Verification items for the finished model (mm, model axes). A direction names the side the tool comes from. Coordinates: 2 decimals unless noted, no trailing zeros. Loops run counter-clockwise (first coordinate to the right, second up) from the corner with the lowest first, then second, coordinate; pieces in that order, holes last. Notation, with made-up numbers: (83, 36.25) -> (137, 36.25) arc R12 cw to (137, 49.25) -> close; hole circle Ø7 at (-3.5, -17.5). An arc over 180 degrees is marked (long way). Use CSV: the item, a comma, the result in double quotes. Start each with the question number.
```python
from build123d import *

# Parameters (mm, degrees)
SKETCH1_R                = 75
BOSS_EXTRUDE1_DEPTH      = 100
SKETCH5_R                = 29
CUT_EXTRUDE2_DEPTH       = 7
BOSS_EXTRUDE2_DEPTH      = 60
BOSS_EXTRUDE2_DEPTH_BACK = 60
SKETCH8_W                = 220
SKETCH8_H                = 180
BOSS_EXTRUDE3_DEPTH      = 10
SKETCH9_R                = 5
CUT_EXTRUDE4_DEPTH       = 10
FILLET1_R                = 10
SKETCH14_R               = 6
CUT_EXTRUDE6_DEPTH       = 110
SKETCH15_R               = 18.5
CUT_EXTRUDE7_DEPTH       = 97
SKETCH16_R               = 1.5
CUT_EXTRUDE8_DEPTH       = 7
SKETCH17_R               = 55
CUT_EXTRUDE9_DEPTH       = 73
SKETCH21_W               = 60
SKETCH21_H               = 80
CUT_EXTRUDE10_DEPTH      = 73
SKETCH23_R               = 2.75
CUT_EXTRUDE11_DEPTH      = 3
CUT_EXTRUDE15_DEPTH      = 40
CUT_EXTRUDE15_DEPTH_BACK = 40


with BuildPart() as part:
    # Sketch1 → Boss-Extrude1 (new body)
    with BuildSketch(Plane(origin=(0, 0, 0), x_dir=(1, 0, 0), z_dir=(0, 1, 0))):
        with Locations(Location((0, 0, 0), (0, 0, 270))):
            Circle(SKETCH1_R)
    extrude(amount=BOSS_EXTRUDE1_DEPTH)

    # Sketch5 → Cut-Extrude2 (cut)
    with BuildSketch(Plane(origin=(0, 100, 0), x_dir=(1, 0, 0), z_dir=(0, 1, 0))):
        with Locations(Location((0, 0, 0), (0, 0, 270))):
            Circle(SKETCH5_R)
    extrude(amount=-CUT_EXTRUDE2_DEPTH, mode=Mode.SUBTRACT)

    # Sketch2 → Boss-Extrude2 (add, two sides: drawn at the far end of the back side and taken through both)
    with BuildSketch(Plane.XY.offset(-BOSS_EXTRUDE2_DEPTH_BACK)):
        Polygon((0, 0), (-125, 0), (-90, 80), (0, 80), align=None)
    extrude(amount=BOSS_EXTRUDE2_DEPTH + BOSS_EXTRUDE2_DEPTH_BACK)

    # Sketch8 → Boss-Extrude3 (add)
    with BuildSketch(Plane.XZ):
        with Locations((-25, 0)):
            Rectangle(SKETCH8_W, SKETCH8_H)
    extrude(amount=BOSS_EXTRUDE3_DEPTH)

    # Sketch9 → Cut-Extrude4 (cut)
    with BuildSketch(Plane.XZ.offset(10)):
        with Locations(Location((-115, 70, 0), (0, 0, 270))):
            Circle(SKETCH9_R)
        with Locations(Location((65, 70, 0), (0, 0, 90))):
            Circle(SKETCH9_R)
        with Locations(Location((65, -70, 0), (0, 0, 270))):
            Circle(SKETCH9_R)
        with Locations(Location((-115, -70, 0), (0, 0, 90))):
            Circle(SKETCH9_R)
    extrude(amount=-CUT_EXTRUDE4_DEPTH, mode=Mode.SUBTRACT)

    # Fillet1
    fillet1_edges = [part.edges().sort_by_distance(p)[0] for p in [
        (-67.5, 80, 60),
        (-107.5, 40, 60),
        (-107.5, 40, -60),
        (-67.5, 80, -60),
        (-90, 80, 0),
    ]]
    fillet(fillet1_edges, radius=FILLET1_R)

    # Sketch14 → Cut-Extrude6 (cut)
    with BuildSketch(Plane(origin=(0, 93, 0), x_dir=(1, 0, 0), z_dir=(0, 1, 0))):
        with Locations(Location((0, 0, 0), (0, 0, 270))):
            Circle(SKETCH14_R)
    extrude(amount=-CUT_EXTRUDE6_DEPTH, mode=Mode.SUBTRACT)

    # Sketch15 → Cut-Extrude7 (cut)
    with BuildSketch(Plane.XZ.offset(10)):
        with Locations(Location((-7, 0, 0), (0, 0, 270))):
            Circle(SKETCH15_R)
    extrude(amount=-CUT_EXTRUDE7_DEPTH, mode=Mode.SUBTRACT)

    # Sketch16 → Cut-Extrude8 (cut)
    with BuildSketch(Plane.XZ.offset(-87)):
        with Locations(Location((-7, 15.5, 0), (0, 0, 270))):
            Circle(SKETCH16_R)
        with Locations(Location((6.423393759, 7.75, 0), (0, 0, 270))):
            Circle(SKETCH16_R)
        with Locations(Location((6.423393759, -7.75, 0), (0, 0, 270))):
            Circle(SKETCH16_R)
        with Locations(Location((-7, -15.5, 0), (0, 0, 270))):
            Circle(SKETCH16_R)
        with Locations(Location((-20.423393759, -7.75, 0), (0, 0, 270))):
            Circle(SKETCH16_R)
        with Locations(Location((-20.423393759, 7.75, 0), (0, 0, 270))):
            Circle(SKETCH16_R)
    extrude(amount=-CUT_EXTRUDE8_DEPTH, mode=Mode.SUBTRACT)

    # Sketch17 → Cut-Extrude9 (cut)
    with BuildSketch(Plane.XZ.offset(10)):
        with Locations(Location((0, 0, 0), (0, 0, 270))):
            Circle(SKETCH17_R)
    extrude(amount=-CUT_EXTRUDE9_DEPTH, mode=Mode.SUBTRACT)

    # Sketch21 → Cut-Extrude10 (cut)
    with BuildSketch(Plane.XZ.offset(10)):
        with Locations((-30, 0)):
            Rectangle(SKETCH21_W, SKETCH21_H)
    extrude(amount=-CUT_EXTRUDE10_DEPTH, mode=Mode.SUBTRACT)

    # Sketch23 → Cut-Extrude11 (cut)
    with BuildSketch(Plane(origin=(0, 93, 0), x_dir=(1, 0, 0), z_dir=(0, 1, 0))):
        with Locations(Location((-7, 15.5, 0), (0, 0, 270))):
            Circle(SKETCH23_R)
        with Locations(Location((6.423393759, 7.75, 0), (0, 0, 270))):
            Circle(SKETCH23_R)
        with Locations(Location((6.423393759, -7.75, 0), (0, 0, 270))):
            Circle(SKETCH23_R)
        with Locations(Location((-7, -15.5, 0), (0, 0, 270))):
            Circle(SKETCH23_R)
        with Locations(Location((-20.423393759, -7.75, 0), (0, 0, 270))):
            Circle(SKETCH23_R)
        with Locations(Location((-20.423393759, 7.75, 0), (0, 0, 270))):
            Circle(SKETCH23_R)
    extrude(amount=-CUT_EXTRUDE11_DEPTH, mode=Mode.SUBTRACT)

    # Sketch27 → Cut-Extrude15 (cut, two sides: drawn at the far end of the back side and taken through both)
    with BuildSketch(Plane.XY.offset(-CUT_EXTRUDE15_DEPTH_BACK)):
        Polygon((-25, -10), (-25, 63), (-74.613551793, 63), (-106.551051793, -10), align=None)
    extrude(amount=CUT_EXTRUDE15_DEPTH + CUT_EXTRUDE15_DEPTH_BACK, mode=Mode.SUBTRACT)


solid = part.part
```
1. Cross-section at C-C, the plane z = -70. Record the boundary of the cut face in (x, y).
2. Cross-section at D-D, the plane x = 65. Record the boundary of the cut face in (y, z).
3. Set-up check for faces 1 (the cylindrical face through (-8.673, 91.521, 13.318)), 2 (the flat face through (-65, 26, 40)), 3 (the flat face through (-51, -10, 41)): record each of +Z, -Z, +X, -X, +Y, -Y from which the full face is reachable in a straight line by a thin tool's end or side.
4. Release check for a two-part mould opening along X. For faces 4 (the flat face through (-7, 87, 0)), 5 (the flat face through (85, -5, -1)), 6 (the cylindrical face through (-105.829, 36.317, 57.148)), 7 (the flat face through (-71, 35, -60)) record: released by +X, released by -X, zero draft, split by the parting line, or undercut.
5. Depth check by flat-ended pin: pin 1 (8 mm diameter, centred on x = 65, z = -70, fed in from +Y); pin 2 (10 mm diameter, centred on x = -101.5, z = -50, fed in from +Y); pin 3 (5 mm diameter, centred on x = 25, y = 41, fed in from +Z); pin 4 (8 mm diameter, centred on x = -71, y = 66, fed in from -Z). Enter the tip coordinate at first touch or a pass-through.
6. Cross-section at A-A, the plane z = 0. Record the boundary of the cut face in (x, y).
7. Cross-section at B-B, the plane x = 0. Record the boundary of the cut face in (y, z), plus the area to 3 significant figures.
8. Scan lines: line 1 (X direction, y = -7, z = -70); line 2 (Z direction, x = 69, y = -4.5); line 3 (Z direction, x = 0, y = 8). Record each from-to range of solid material in increasing order.
Solution:
1,outline,"(-135, -10) -> (-120, -10) -> (-120, 0) -> (-135, 0) -> close; (-110, -10) -> (60, -10) -> (60, 0) -> (26.93, 0) -> (26.93, 100) -> (-26.93, 100) -> (-26.93, 0) -> (-110, 0) -> close; (70, -10) -> (85, -10) -> (85, 0) -> (70, 0) -> close"
2,outline,"(-10, -90) -> (0, -90) -> (0, -75) -> (-10, -75) -> close; (-10, -65) -> (0, -65) -> (0, -37.42) -> (100, -37.42) -> (100, 37.42) -> (0, 37.42) -> (0, 65) -> (-10, 65) -> close; (-10, 75) -> (0, 75) -> (0, 90) -> (-10, 90) -> close"
3,face 1,"+Y"
3,face 2,"-Y"
3,face 3,"+Z, -Z, +X, -X, -Y"
4,face 4,"undercut"
4,face 5,"released by +X"
4,face 6,"released by -X"
4,face 7,"zero draft"
5,pin 1,"passes through"
5,pin 2,"stops at y = 65.14"
5,pin 3,"stops at z = 71.55"
5,pin 4,"stops at z = -60"
6,outline,"(-135, -10) -> (-106.55, -10) -> (-74.61, 63) -> (-25.5, 63) -> (-25.5, 87) -> (-6, 87) -> (-6, 93) -> (-29, 93) -> (-29, 100) -> (-75, 100) -> (-75, 80) -> (-83.46, 80) arc R10 ccw to (-92.62, 74.01) -> (-125, 0) -> (-135, 0) -> close; (6, 87) -> (11.5, 87) -> (11.5, 63) -> (55, 63) -> (55, -10) -> (85, -10) -> (85, 0) -> (75, 0) -> (75, 100) -> (29, 100) -> (29, 93) -> (6, 93) -> close"
7,outline,"(-10, -90) -> (0, -90) -> (0, -75) -> (100, -75) -> (100, -29) -> (93, -29) -> (93, -6) -> (87, -6) -> (87, -17.12) -> (63, -17.12) -> (63, -55) -> (-10, -55) -> close; (-10, 55) -> (63, 55) -> (63, 17.12) -> (87, 17.12) -> (87, 6) -> (93, 6) -> (93, 29) -> (100, 29) -> (100, 75) -> (0, 75) -> (0, 90) -> (-10, 90) -> close"
7,area,"7,470 mm2"
8,line 1,"x = -135 to -120, -110 to 60, 70 to 85"
8,line 2,"z = -90 to -73, -67 to 67, 73 to 90"
8,line 3,"z = -75 to -55, 55 to 75"
